```python
from build123d import *

# Parameters (mm, degrees)
CYLINDER1709_R     = 1.5
CYLINDER1709_DEPTH = 60
CYLINDER1710_R     = 1.5
CYLINDER1710_DEPTH = 60
CYLINDER1702_R     = 1.5
CYLINDER1702_DEPTH = 60
CYLINDER1706_R     = 1.5
CYLINDER1706_DEPTH = 60
CYLINDER1703_R     = 2.5
CYLINDER1703_DEPTH = 48
BOX666_W           = 28.8
BOX666_H           = 34.21
BOX666_DEPTH       = 20
BOX665_W           = 42
BOX665_H           = 20
BOX665_DEPTH       = 24
CHAMFER053_SIZE    = 6
CHAMFER054_SIZE    = 4
CHAMFER056_SIZE    = 2


with BuildPart() as obj1:
    # Cylinder1709 → Cylinder1709 (new body)
    with BuildSketch(Plane(origin=(18, 85, -57), x_dir=(1, 0, 0), z_dir=(0, 0, 1))):
        Circle(CYLINDER1709_R)
    extrude(amount=CYLINDER1709_DEPTH)


with BuildPart() as obj2:
    # Cylinder1710 → Cylinder1710 (new body)
    with BuildSketch(Plane(origin=(-18, 85, -57), x_dir=(1, 0, 0), z_dir=(0, 0, 1))):
        Circle(CYLINDER1710_R)
    extrude(amount=CYLINDER1710_DEPTH)


with BuildPart() as obj3:
    # Cylinder1702 → Cylinder1702 (new body)
    with BuildSketch(Plane(origin=(-18, 95, -57), x_dir=(1, 0, 0), z_dir=(0, 0, 1))):
        Circle(CYLINDER1702_R)
    extrude(amount=CYLINDER1702_DEPTH)


with BuildPart() as compound850:
    # Cylinder1706 → Cylinder1706 (new body)
    with BuildSketch(Plane(origin=(18, 95, -57), x_dir=(1, 0, 0), z_dir=(0, 0, 1))):
        Circle(CYLINDER1706_R)
    extrude(amount=CYLINDER1706_DEPTH)

    # Compound850: union obj1, obj2, obj3
    add(obj1.part)
    add(obj2.part)
    add(obj3.part)


with BuildPart() as compound850_1:
    # Compound850 placement: moved
    add(compound850.part.moved(Location((0, 0, -16))))


with BuildPart() as obj4:
    # Cylinder1703 → Cylinder1703 (new body)
    with BuildSketch(Plane(origin=(0, 90, -55), x_dir=(1, 0, 0), z_dir=(0, 0, 1))):
        Circle(CYLINDER1703_R)
    extrude(amount=CYLINDER1703_DEPTH)


with BuildPart() as compound846:
    # Box666 → Box666 (new body)
    with BuildSketch(Plane(origin=(-14.4, -15.34, 34), x_dir=(1, 0, 0), z_dir=(0, 0, 1))):
        with Locations((14.4, 17.105)):
            Rectangle(BOX666_W, BOX666_H)
    extrude(amount=BOX666_DEPTH)


with BuildPart() as compound846_1:
    # Compound846 placement: moved
    add(compound846.part.moved(Location((0, 90, -83))))


with BuildPart() as chamfer056:
    # Box665 → Box665 (new body)
    with BuildSketch(Plane(origin=(-21, 80, -49), x_dir=(1, 0, 0), z_dir=(0, 0, 1))):
        with Locations((21, 10)):
            Rectangle(BOX665_W, BOX665_H)
    extrude(amount=BOX665_DEPTH)

    # Cut354: cut Compound846
    add(compound846_1.part, mode=Mode.SUBTRACT)


with BuildPart() as chamfer056_1:
    # Cut354 placement: moved
    add(chamfer056.part.moved(Location((0, 0, 21))))

    # Cut352: cut obj4
    add(obj4.part, mode=Mode.SUBTRACT)

    # Chamfer053
    chamfer053_edges = [chamfer056_1.edges().sort_by_distance(p)[0] for p in [
        (-14.4, 80, -18),
        (14.4, 80, -18),
    ]]
    chamfer(chamfer053_edges, length=CHAMFER053_SIZE)

    # Cut348: cut Compound850
    add(compound850_1.part, mode=Mode.SUBTRACT)

    # Chamfer054
    chamfer054_edges = [chamfer056_1.edges().sort_by_distance(p)[0] for p in [
        (-21, 90, -4),
        (21, 90, -4),
    ]]
    chamfer(chamfer054_edges, length=CHAMFER054_SIZE)

    # Chamfer056
    chamfer056_edges = [chamfer056_1.edges().sort_by_distance(p)[0] for p in [
        (-21, 100, -18),
        (21, 100, -18),
    ]]
    chamfer(chamfer056_edges, length=CHAMFER056_SIZE)


solid = chamfer056_1.part
```
For this review, take the finished solid that the model builds, in its own axes (mm). A direction names the side the tool comes from. Round coordinates to 2 decimals unless told otherwise and drop trailing zeros. Order: outer loops, then holes, each group sorted by start corner. A loop starts at its lowest first (then second) coordinate and runs counter-clockwise, first axis right, second up.
Q1. We need section D-D, the plane z = -6.5. Give the boundary of the cut face in (x, y).
Findings below:
outline: (-19.5, 80) - (19.5, 80) - (19.5, 99.5) - (19, 100) - (-19, 100) - (-19.5, 99.5) - close
Q2. Mouldability with a two-part tool opening along Y and no side actions: class faces 5 (the cylindrical face through (-0.33, 92.48, -7.51)), 6 (the flat face through (20, 99, -17)), 7 (the flat face through (-17.4, 83, -18.1)), 8 (the flat face through (14.4, 93, -18)) as pulls with the +Y half, pulls with the -Y half, needs draft (parallel to the pull), parting line crosses it, or undercut.
Findings below:
face 5: undercut
face 6: pulls with the +Y half
face 7: pulls with the -Y half
face 8: needs draft
Q3. We need section A-A, the plane z = -22.25. Give the boundary of the cut face in (x, y), plus the area to 3 significant figures.
Findings below:
outline: (-21, 80) - (-20.4, 80) - (-14.4, 86) - (-14.4, 100) - (-19, 100) - (-21, 98) - close; (14.4, 86) - (20.4, 80) - (21, 80) - (21, 98) - (19, 100) - (14.4, 100) - close; hole circle Ø3 at (-18, 85); hole circle Ø3 at (-18, 95); hole circle Ø3 at (18, 85); hole circle Ø3 at (18, 95)
area: 196 mm2
Q4. Insertion check: P1, Ø1.5, axis at x = -14, z = -19.5, coming from the -Y side; P2, Ø0.9, axis at x = 18, y = 94.5, coming from the -Z side; P3, Ø6.5, axis at x = 0, y = 90, coming from the -Z side; P4, Ø10, axis at x = -7, z = -23, coming from the -Y side. Each pin has a flat end and moves straight along its axis. Give the tip position at first contact, or say it passes through.
Findings below:
P1: stops at y = 85.65
P2: stops at z = -13
P3: stops at z = -8
P4: passes through
Q5. Wall thickness on line 1 (X direction, y = 95, z = -20); line 2 (X direction, y = 91, z = -25.5); line 3 (Y direction, x = -18, z = -21.25): over which ranges is each line inside the solid? List them lowest first.
Findings below:
line 1: x = -21 to -19.5, -16.5 to -14.4, 14.4 to 16.5, 19.5 to 21
line 2: x = -21 to -14.4, 14.4 to 21
line 3: y = 82.4 to 83.5, 86.5 to 93.5, 96.5 to 100
Q6. We need section C-C, the plane x = 0. Give the boundary of the cut face in (y, z), plus the area to 3 significant figures.
Findings below:
outline: (80, -8) - (87.5, -8) - (87.5, -7) - (92.5, -7) - (92.5, -8) - (100, -8) - (100, -4) - (80, -4) - close
area: 75.0 mm2
Q7. We need section B-B, the plane y = 90. Give the boundary of the cut face in (x, z).
Findings below:
outline: (-21, -28) - (-14.4, -28) - (-14.4, -8) - (-2.5, -8) - (-2.5, -7) - (2.5, -7) - (2.5, -8) - (14.4, -8) - (14.4, -28) - (21, -28) - (21, -8) - (17, -4) - (-17, -4) - (-21, -8) - close
Q8. Machinability: for faces 1 (the flat face through (17.4, 83, -18.1)), 2 (the flat face through (0, 90, -7)), 3 (the flat face through (-14.4, 93, -18)), 4 (the flat face through (-19, 90, -6)), which of the approach directions +Z, -Z, +X, -X, +Y, -Y give a long, thin tool a straight path to every point of the face, cutting with its end or side? Answer none if there is none.
Findings below:
face 1: -Z, -Y
face 2: -Z
face 3: -Z, +Y, -Y
face 4: +Z, -X, +Y, -Y
